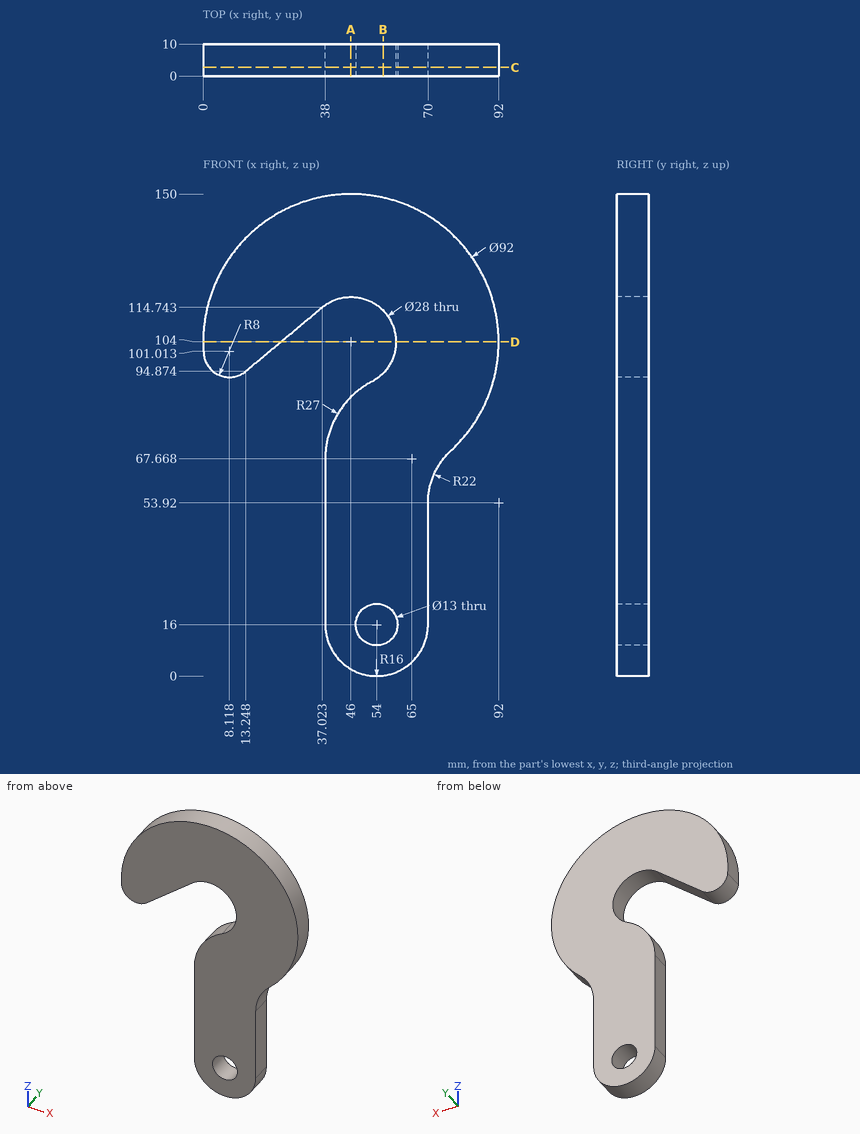
Could you check a few things on this drawing? It's one solid part, dimensions in mm from its lowest x, y, z. Round coordinates to 2 decimals unless told otherwise and drop trailing zeros. Write each loop counter-clockwise with the first axis right and the second up, starting at its lowest first coordinate (ties: lowest second). Pieces come first, ordered by that corner, then holes. Notation, with made-up numbers: M 72.5,50 L 128.5,50 A21 cw 128.5,88 Z; hole C -7,56 d7. An arc over 180 degrees is marked long. Answer as CSV lines item,"result". Start each with the question number.
1. Suppose I cut it at A-A on x = 46. Write out the boundary of the cut face in (y, z).
2. Suppose I cut it at C-C on y = 2.75. Write out the boundary of the cut face in (x, z) (1 decimal).
3. Suppose I cut it at B-B on x = 56. Write out the boundary of the cut face in (y, z) (1 decimal), then the cut area to 3 significant figures.
4. I need wall thicknesses on probe 1 along X at (y, z) = (2.5, 16.5); probe 2 along Z at (x, y) = (53, 6.5) (1 decimal); probe 3 along X at (y, z) = (4, 17). Which ranges of each line are inside material? Lowest first, please.
5. I'm going to push flat-ended pins straight in: pin 1 Ø5 at (y, z) = (4, 36) entering from -X; pin 2 Ø2 at (y, z) = (2, 107) entering from -X; pin 3 Ø6 at (x, y) = (69.5, 8.5) entering from -Z. Where does each tip first touch, or does it pass through?
6. Suppose I cut it at D-D on z = 104. Write out the boundary of the cut face in (x, y), then the cut area to 3 significant figures.
Check result:
1,outline,"M 0,2.14 L 10,2.14 L 10,86.85 L 0,86.85 Z; M 0,118 L 10,118 L 10,150 L 0,150 Z"
2,outline,"M 0.1,100.4 A8 ccw 13.2,94.9 L 37,114.7 A14 cw long 52.5,91.6 A27 ccw 38,67.7 L 38,16 A16 ccw 70,16 L 70,53.9 A22 cw 77.1,70.1 A46 ccw long Z; hole C 54,16 d13"
3,outline,"M 0,0.1 L 10,0.1 L 10,9.8 L 0,9.8 Z; M 0,22.2 L 10,22.2 L 10,94.2 L 0,94.2 Z; M 0,113.8 L 10,113.8 L 10,148.9 L 0,148.9 Z"
3,area,"1,170 mm2"
4,probe 1,"x = 38 to 47.52, 60.48 to 70"
4,probe 2,"z = 0 to 9.6, 22.4 to 91.9, 116.1 to 149.5"
4,probe 3,"x = 38 to 47.58, 60.42 to 70"
5,pin 1,"stops at x = 38"
5,pin 2,"stops at x = 0.04"
5,pin 3,"stops at z = 6.01"
6,outline,"M 0,0 L 24.17,0 L 24.17,10 L 0,10 Z; M 60,0 L 92,0 L 92,10 L 60,10 Z"
6,area,"562 mm2"
